from build123d import *

# Parameters (mm, degrees)
F0_R      = 25.4
F1_DEPTH  = 1.5875
F2_R      = 26.19375
F3_DEPTH  = 3.175
F4_R      = 26.19375
F5_DEPTH  = 3.175
F7_DEPTH  = 38.1
F9_DEPTH  = 6.35
F10_R     = 1.651
F11_DEPTH = 25.4


with BuildPart() as f1:
    # F0 (on Front) → F1 (new body, symmetric)
    with BuildSketch(Plane.XZ):
        Circle(F0_R)
    extrude(amount=F1_DEPTH, both=True)

    # F2 (on face) → F3 (join)
    with BuildSketch(Plane.XZ.offset(1.5875)):
        Circle(F2_R)
    extrude(amount=F3_DEPTH)

    # F4 (on face) → F5 (join)
    with BuildSketch(Plane(origin=(0, 1.5875, 0), x_dir=(-1, 0, 0), z_dir=(0, 1, 0))):
        Circle(F4_R)
    extrude(amount=F5_DEPTH)

    # F6 (on face) → F7 (cut, symmetric)
    with BuildSketch(Plane(origin=(0, 4.7625, 0), x_dir=(-1, 0, 0), z_dir=(0, 1, 0))):
        with BuildLine():
            ThreePointArc((-17.552633, -11.419258), (-10.090636, -18.630629), (0, -21.052268))
            ThreePointArc((0, -21.052268), (4.445, -16.607268), (0, -12.162268))
            ThreePointArc((0, -12.162268), (-5.690238, -10.297309), (-10.319898, -6.49953))
            ThreePointArc((-10.319898, -6.49953), (-16.882294, -4.628293), (-17.552633, -11.419258))
        make_face()
        with BuildLine():
            ThreePointArc((10.231966, 6.712214), (11.485159, 0.501891), (10.718335, -5.787035))
            ThreePointArc((10.718335, -5.787035), (10.366031, -6.884623), (9.950625, -7.959916))
            ThreePointArc((9.950625, -7.959916), (13.047399, -12.543448), (18.211526, -10.560884))
            ThreePointArc((18.211526, -10.560884), (21.619656, -0.962225), (18.79669, 8.824525))
            ThreePointArc((18.79669, 8.824525), (13.317942, 12.619318), (10.231966, 6.712214))
        make_face()
        with BuildLine():
            ThreePointArc((-10.721463, 5.782488), (-5.701405, 9.544893), (0, 12.162268))
            ThreePointArc((0, 12.162268), (4.445, 16.607268), (0, 21.052268))
            ThreePointArc((0, 21.052268), (-1.096134, 20.782721), (-2.183325, 20.479104))
            ThreePointArc((-2.183325, 20.479104), (-10.013079, 17.11314), (-16.838004, 12.008714))
            ThreePointArc((-16.838004, 12.008714), (-17.468207, 11.394684), (-18.083289, 10.765508))
            ThreePointArc((-18.083289, 10.765508), (-17.523515, 5.158655), (-11.915992, 4.605625))
            ThreePointArc((-11.915992, 4.605625), (-11.32708, 5.202535), (-10.721463, 5.782488))
        make_face()
    extrude(amount=F7_DEPTH, both=True, mode=Mode.SUBTRACT)

    # F8 (on face) → F9 (cut)
    with BuildSketch(Plane.XZ.offset(4.7625)):
        Polygon((2.611876, -6.851382), (7.239409, -1.16374), (4.627533, 5.687642), (-2.611876, 6.851382), (-7.239409, 1.16374), (-4.627533, -5.687642), align=None)
    extrude(amount=-F9_DEPTH, mode=Mode.SUBTRACT)

    # F10 (on face) → F11 (cut)
    with BuildSketch(Plane(origin=(0, 4.7625, 0), x_dir=(-1, 0, 0), z_dir=(0, 1, 0))):
        Circle(F10_R)
    extrude(amount=-F11_DEPTH, mode=Mode.SUBTRACT)


solid = f1.part
Input: part model. Units: mm. Frame: model coordinates. A direction names the side the tool comes from. Round coordinates to 2 decimals unless told otherwise and drop trailing zeros. Write each loop counter-clockwise with the first axis right and the second up, starting at its lowest first coordinate (ties: lowest second). Pieces come first, ordered by that corner, then holes.
1) Cut plane D-D (y = -3). Return the cut outline in (x, z) (1 decimal), then the cut area to 3 significant figures.
2) Ray query, L1, parallel to X at y = 1.75, z = -0.5; L2, parallel to Z at x = -4, y = 1.75; L3, parallel to Z at x = -4, y = -1. Return the intervals inside material, ascending.
3) Contact query for flat-ended pins moving along their axis: P1, Ø1.5, axis at x = -7, y = 1, coming from the -Z side; P2, Ø1, axis at y = -3.5, z = -20.5, coming from the +X side; P3, Ø3, axis at x = -19.5, z = 2, coming from the +Y side; P4, Ø5, axis at y = 0.5, z = -4, coming from the +X side. Output: stop coordinate, or through.
4) Cut plane B-B (x = -13.5). Return the cut outline in (y, z).
5) Reachability of faces 4 (the flat face through (4.89, -1.63, -4.05)), 5 (the cylindrical face through (5.78, 0.07, 9.5)), 6 (the flat face through (-25.3, -1.588, 4)) from +Z, -Z, +X, -X, +Y, -Y: full face, straight path, thin tool, end or side. Return the list, or none.
6) Cut plane A-A (y = 3). Return the cut outline in (x, z) (1 decimal), then the cut area to 3 significant figures.
7) Draft query along Z for faces 1 (the cylindrical face through (-4.444, 0.067, 16.51)), 2 (the cylindrical face through (-5.506, -0.022, -24.796)), 3 (the flat face through (25.3, 1.588, 4)). Return one class per face: pulls with the +Z half, pulls with the -Z half, needs draft (parallel to the pull), parting line crosses it, or undercut.
8) Cut plane C-C (z = -9). Return the cut outline in (x, y), then the cut area to 3 significant figures.
Geometry says:
1. outline: circle Ø52.4 at (0, 0); hole (-18.8, 8.8) arc R16.6 ccw to (-18.2, -10.6) arc R4.4 ccw to (-10, -8) arc R19.9 cw to (-10.7, -5.8) arc R19.9 cw to (-10.2, 6.7) arc R4.4 ccw (long way) to start; hole (-7.2, 1.2) - (-4.6, -5.7) - (2.6, -6.9) - (7.2, -1.2) - (4.6, 5.7) - (-2.6, 6.9) - close; hole (0, -21.1) arc R19.7 ccw to (17.6, -11.4) arc R4.4 ccw (long way) to (10.3, -6.5) arc R16.3 cw to (0, -12.2) arc R4.4 ccw to start; hole (0, 12.2) arc R29.5 cw to (10.7, 5.8) arc R29.5 cw to (11.9, 4.6) arc R4.4 ccw to (18.1, 10.8) arc R36.2 ccw to (16.8, 12) arc R36.2 ccw to (2.2, 20.5) arc R36.2 ccw to (0, 21.1) arc R4.4 ccw to start
1. area: 1,360 mm2
2. L1: x = -26.19 to -21.63, -11.5 to -1.57, 1.57 to 26.19
2. L2: z = -25.89 to -18.55, -14.67 to 14.67, 18.55 to 25.89
2. L3: z = -25.08 to -18.55, -14.67 to -5.79, 5.15 to 14.67, 18.55 to 25.08
3. P1: stops at z = -25.37
3. P2: stops at x = 16.91
3. P3: passes through
3. P4: stops at x = 26.14
4. outline: (-4.76, -22.45) - (-1.59, -22.45) - (-1.59, -21.52) - (1.59, -21.52) - (1.59, -22.45) - (4.76, -22.45) - (4.76, -12.66) - (-4.76, -12.66) - close; (-4.76, 12.66) - (4.76, 12.66) - (4.76, 22.45) - (1.59, 22.45) - (1.59, 21.52) - (-1.59, 21.52) - (-1.59, 22.45) - (-4.76, 22.45) - close
5. face 4: -Y
5. face 5: +Y, -Y
5. face 6: none
6. outline: circle Ø52.4 at (0, 0); hole (-18.8, 8.8) arc R16.6 ccw to (-18.2, -10.6) arc R4.4 ccw to (-10, -8) arc R19.9 cw to (-10.7, -5.8) arc R19.9 cw to (-10.2, 6.7) arc R4.4 ccw (long way) to start; hole circle Ø3.3 at (0, 0); hole (0, -21.1) arc R19.7 ccw to (17.6, -11.4) arc R4.4 ccw (long way) to (10.3, -6.5) arc R16.3 cw to (0, -12.2) arc R4.4 ccw to start; hole (0, 12.2) arc R29.5 cw to (10.7, 5.8) arc R29.5 cw to (11.9, 4.6) arc R4.4 ccw to (18.1, 10.8) arc R36.2 ccw to (16.8, 12) arc R36.2 ccw to (2.2, 20.5) arc R36.2 ccw to (0, 21.1) arc R4.4 ccw to start
6. area: 1,490 mm2
7. face 1: undercut
7. face 2: parting line crosses it
7. face 3: needs draft
8. outline: (-24.6, -4.76) - (-19.27, -4.76) - (-19.27, 4.76) - (-24.6, 4.76) - (-24.6, 1.59) - (-23.75, 1.59) - (-23.75, -1.59) - (-24.6, -1.59) - close; (-9.99, -4.76) - (7.69, -4.76) - (7.69, 4.76) - (-9.99, 4.76) - close; (18.77, -4.76) - (24.6, -4.76) - (24.6, -1.59) - (23.75, -1.59) - (23.75, 1.59) - (24.6, 1.59) - (24.6, 4.76) - (18.77, 4.76) - close
8. area: 269 mm2
